from build123d import *

# Parameters (mm, degrees)
F0_R           = 57.5
F1_DEPTH       = 40
F2_R           = 55
F3_DEPTH       = 35
F4_R           = 3
F5_R           = 2
F6_R           = 12.5
F7_DEPTH       = 40.001
F9_D           = 15
F9_CBORE_D     = 20
F9_CBORE_DEPTH = 0.5
F10_C1_SIZE2   = 2
F10_C1_SIZE    = 0.3526539614
F10_C2_SIZE2   = 0.3526539614
F10_C2_SIZE    = 2
F10_C3_SIZE2   = 0.3526539614
F10_C3_SIZE    = 2
F10_C4_SIZE2   = 0.3526539614
F10_C4_SIZE    = 2
F10_C5_SIZE2   = 0.3526539614
F10_C5_SIZE    = 2
F10_C6_SIZE2   = 0.3526539614
F10_C6_SIZE    = 2
F10_C7_SIZE2   = 0.3526539614
F10_C7_SIZE    = 2
F10_C8_SIZE2   = 0.3526539614
F10_C8_SIZE    = 2
F11_W          = 23.2258066535
F11_H          = 27.9435478151
F11_W_2        = 23.7701628357
F11_H_2        = 28.1250029802
F12_DEPTH      = 57.5010001
F12_DEPTH_BACK = 57.5010001


with BuildPart() as f1:
    # F0 (on Top) → F1 (new body)
    with BuildSketch(Plane.XY):
        Circle(F0_R)
    extrude(amount=F1_DEPTH)

    # F2 (on face) → F3 (cut)
    with BuildSketch(Plane.XY.offset(40)):
        Circle(F2_R)
    extrude(amount=-F3_DEPTH, mode=Mode.SUBTRACT)

    # F4
    f4_edges = [f1.edges().sort_by_distance(p)[0] for p in [
        (-55, 0, 5),
    ]]
    fillet(f4_edges, radius=F4_R)

    # F5
    f5_edges = [f1.edges().sort_by_distance(p)[0] for p in [
        (-57.5, 0, 0),
    ]]
    fillet(f5_edges, radius=F5_R)

    # F6 (on face) → F7 (cut, through all)
    with BuildSketch(Plane(origin=(0, 0, 0), x_dir=(1, 0, 0), z_dir=(0, 0, -1))):
        Circle(F6_R)
    extrude(amount=-F7_DEPTH, mode=Mode.SUBTRACT)

    # F9 (through all)
    with Locations(Plane(origin=(0, 0, 0), x_dir=(1, 0, 0), z_dir=(0, 0, -1))):
        with Locations((-37.5, 0), (-23.3808675697, 29.3186805926), (8.3445350234, 36.5597967068), (33.7863325463, 16.2706402169), (33.7863325463, -16.2706402169), (8.3445350234, -36.5597967068), (-23.3808675697, -29.3186805926)):
            CounterBoreHole(F9_D / 2, F9_CBORE_D / 2, F9_CBORE_DEPTH)

    # F10: chamfer of 2 x 0.3526539614 on 8 edges, made by hand

    # F10_c1
    f10_c1_edges = [f1.edges().sort_by_distance(p)[0] for p in [
        (-12.5, 0, 5),
    ]]
    f10_c1_side = f1.faces().sort_by_distance((-12.5, 0, 4.9929469208))[0]
    chamfer(f10_c1_edges, length=F10_C1_SIZE, length2=F10_C1_SIZE2, reference=f10_c1_side)

    # F10_c2
    f10_c2_edges = [f1.edges().sort_by_distance(p)[0] for p in [
        (-30.8808675697, -29.3186805926, 5),
    ]]
    f10_c2_side = f1.faces().sort_by_distance((-30.8879206489, -29.3186805926, 5))[0]
    chamfer(f10_c2_edges, length=F10_C2_SIZE, length2=F10_C2_SIZE2, reference=f10_c2_side)

    # F10_c3
    f10_c3_edges = [f1.edges().sort_by_distance(p)[0] for p in [
        (0.8445350234, -36.5597967068, 5),
    ]]
    f10_c3_side = f1.faces().sort_by_distance((0.8374819441, -36.5597967068, 5))[0]
    chamfer(f10_c3_edges, length=F10_C3_SIZE, length2=F10_C3_SIZE2, reference=f10_c3_side)

    # F10_c4
    f10_c4_edges = [f1.edges().sort_by_distance(p)[0] for p in [
        (26.2863325463, -16.2706402169, 5),
    ]]
    f10_c4_side = f1.faces().sort_by_distance((26.2792794671, -16.2706402169, 5))[0]
    chamfer(f10_c4_edges, length=F10_C4_SIZE, length2=F10_C4_SIZE2, reference=f10_c4_side)

    # F10_c5
    f10_c5_edges = [f1.edges().sort_by_distance(p)[0] for p in [
        (-45, 0, 5),
    ]]
    f10_c5_side = f1.faces().sort_by_distance((-45.0070530792, 0, 5))[0]
    chamfer(f10_c5_edges, length=F10_C5_SIZE, length2=F10_C5_SIZE2, reference=f10_c5_side)

    # F10_c6
    f10_c6_edges = [f1.edges().sort_by_distance(p)[0] for p in [
        (-30.8808675697, 29.3186805926, 5),
    ]]
    f10_c6_side = f1.faces().sort_by_distance((-30.8879206489, 29.3186805926, 5))[0]
    chamfer(f10_c6_edges, length=F10_C6_SIZE, length2=F10_C6_SIZE2, reference=f10_c6_side)

    # F10_c7
    f10_c7_edges = [f1.edges().sort_by_distance(p)[0] for p in [
        (26.2863325463, 16.2706402169, 5),
    ]]
    f10_c7_side = f1.faces().sort_by_distance((26.2792794671, 16.2706402169, 5))[0]
    chamfer(f10_c7_edges, length=F10_C7_SIZE, length2=F10_C7_SIZE2, reference=f10_c7_side)

    # F10_c8
    f10_c8_edges = [f1.edges().sort_by_distance(p)[0] for p in [
        (0.8445350234, 36.5597967068, 5),
    ]]
    f10_c8_side = f1.faces().sort_by_distance((0.8374819441, 36.5597967068, 5))[0]
    chamfer(f10_c8_edges, length=F10_C8_SIZE, length2=F10_C8_SIZE2, reference=f10_c8_side)

    # F11 (on Front) → F12 (cut, two sides)
    with BuildSketch(Plane.XZ) as f12_sk:
        with Locations((-33.4778241813, 32.3891136795)):
            Rectangle(F11_W, F11_H)
        with Locations((34.4758061692, 32.4798412621)):
            Rectangle(F11_W_2, F11_H_2)
    extrude(amount=F12_DEPTH, mode=Mode.SUBTRACT)
    extrude(f12_sk.sketch, amount=-F12_DEPTH_BACK, mode=Mode.SUBTRACT)


solid = f1.part
Here's how the part is built. I have some questions about the finished solid (model axes, mm). A direction names the side the tool comes from. Round coordinates to 2 decimals unless told otherwise and drop trailing zeros. Loops run counter-clockwise (first coordinate to the right, second up) from the corner with the lowest first, then second, coordinate; pieces in that order, holes last.
1. If we section it at D-D on z = 10.5: Write out the boundary of the cut face in (x, y), plus the area to 3 significant figures.
Answer list:
outline: circle Ø115 at (0, 0); hole circle Ø110 at (0, 0)
area: 884 mm2
2. For P1, Ø6, axis at x = -19, y = 25, coming from the -Z side; P2, Ø18.5, axis at x = 38.5, y = -44.5, coming from the +Z side; P3, Ø8, axis at y = 27.5, z = 9.5, coming from the +X side, each with a flat end and sliding along its axis, tell me the tip position at first contact or that it passes through.
Answer list:
P1: stops at z = 0.5
P2: stops at z = 18.42
P3: stops at x = 52.48
3. If we section it at A-A on z = 33: Write out the boundary of the cut face in (x, y), plus the area to 3 significant figures.
Answer list:
outline: (-45.09, -35.68) - (-45.09, -31.49) arc R55 cw to (-45.09, 31.49) - (-45.09, 35.68) arc R57.5 ccw to start; (-21.86, -53.18) arc R57.5 ccw to (22.59, -52.88) - (22.59, -50.15) arc R55 cw to (-21.86, -50.47) - close; (-21.86, 50.47) arc R55 cw to (22.59, 50.15) - (22.59, 52.88) arc R57.5 ccw to (-21.86, 53.18) - close; (46.36, -34.01) arc R57.5 ccw to (46.36, 34.01) - (46.36, 29.59) arc R55 cw to (46.36, -29.59) - close
area: 578 mm2
4. We'd pull the mould along Y, two halves only. Please class faces 4 (the face through (-45.091, 34, 29)), 5 (the face through (0.974, -43.318, 0.246)), 6 (the face through (-12.465, -56.133, 20.734)): +Y half, -Y half, draft (parallel to the pull), parting line (faces both ways), or undercut.
Answer list:
face 4: draft
face 5: undercut
face 6: parting line
5. If I drill on line 1 along X through (y, z) = (0, 3.55); line 2 along Z through (x, y) = (42, -27.5); line 3 along X through (y, z) = (37, 15), over which ranges is the centre line in solid material (lowest first)?
Answer list:
line 1: x = -57.5 to -45, -30 to -12.5, 12.5 to 57.5
line 2: z = 0 to 5
line 3: x = -44.01 to -40.69, 40.69 to 44.01
6. Which directions (+Z, -Z, +X, -X, +Y, -Y) give clear straight access to the entire face, cutting with the end or side of a thin tool? Please do faces 1 (the face through (31.5, 8.8, 0.5)), 2 (the face through (22.591, 51, 29)), 3 (the face through (46.361, 32, 29)).
Answer list:
face 1: -Z
face 2: +Z, +X, +Y, -Y
face 3: +Z, +Y, -Y
7. If we section it at C-C on x = 34.5: Count the separate pieces of the cut face and the enclosed holes in it, plus the area to 3 significant figures.
Answer list:
separate pieces: 3
enclosed holes: 0
area: 392 mm2
8. If we section it at B-B on y = 0: Write out the boundary of the cut face in (x, z).
Answer list:
outline: (-57.5, 2) arc R2 ccw to (-55.5, 0) - (-47.5, 0) - (-47.5, 0.5) - (-45, 0.5) - (-45, 4.65) - (-47, 5) - (-52, 5) arc R3 cw to (-55, 8) - (-55, 40) - (-57.5, 40) - close; (-30, 0.5) - (-27.5, 0.5) - (-27.5, 0) - (-12.5, 0) - (-12.5, 4.65) - (-14.5, 5) - (-28, 5) - (-30, 4.65) - close; (12.5, 0) - (55.5, 0) arc R2 ccw to (57.5, 2) - (57.5, 40) - (55, 40) - (55, 8) arc R3 cw to (52, 5) - (14.5, 5) - (12.5, 4.65) - close
